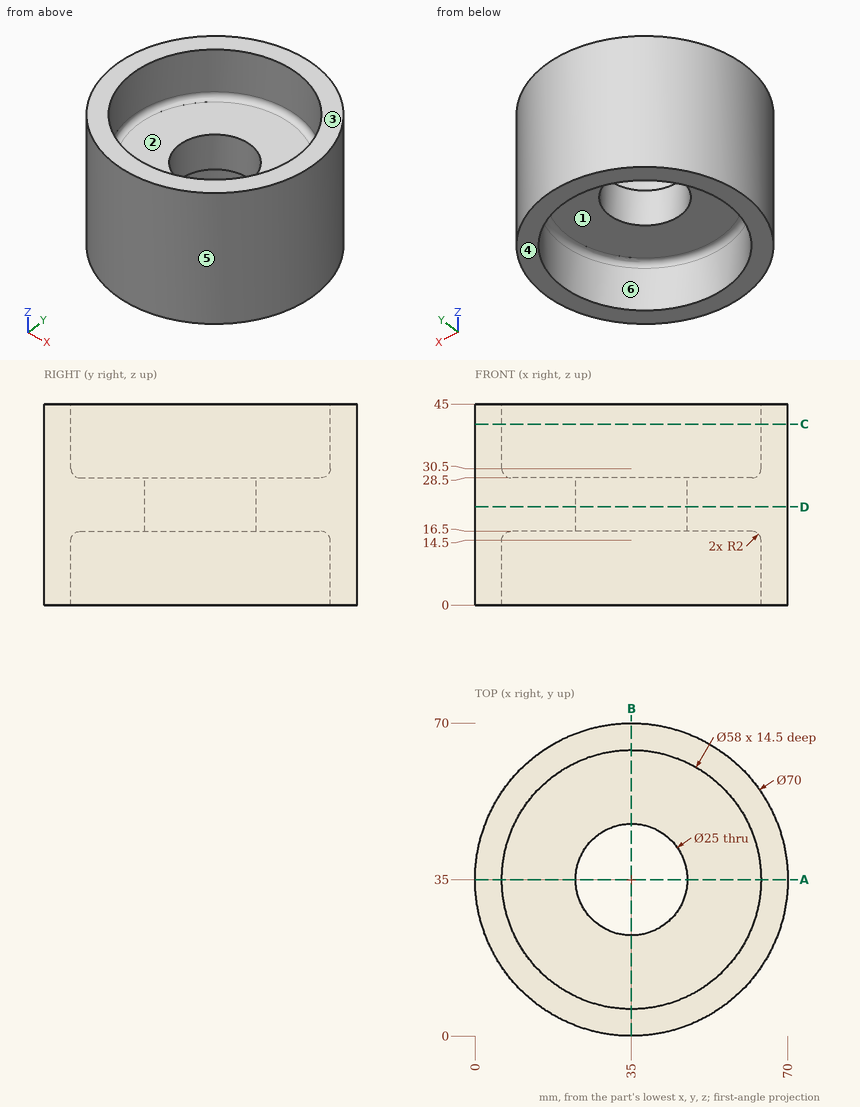
Could you check a few things on this drawing? It's one solid part, dimensions in mm from its lowest x, y, z. A direction names the side the tool comes from. Round coordinates to 2 decimals unless told otherwise and drop trailing zeros. Order: outer loops, then holes, each group sorted by start corner. A loop starts at its lowest first (then second) coordinate and runs counter-clockwise, first axis right, second up. Notation, with made-up numbers: M 82,46 L 115,46 A29 ccw 115,84 Z; hole C 59,-28.5 d6. An arc over 180 degrees is marked long. One line per question, with ' | ' between items. Start each with the question number.
(1) For P1, Ø10, axis at y = 19, z = 37, coming from the -X side; P2, Ø1, axis at x = 59.5, y = 31.5, coming from the -Z side; P3, Ø8, axis at y = 11, z = 8.5, coming from the +X side; P4, Ø3, axis at x = 46.5, y = 8.5, coming from the +Z side, each with a flat end and sliding along its axis, tell me the tip position at first contact or that it passes through.
(2) Suppose I cut it at D-D on z = 22. List the corners of the cut face in (x, y) for me, then the cut area to 3 significant figures.
(3) For the marked faces 1, 2 and 3, which set-ups out of +Z, -Z, +X, -X, +Y, -Y let a thin tool reach every point of the face, with its end or its side?
(4) Please list where these lines run through material, in increasing order: line 1 along Y through (x, z) = (35, 36); line 2 along X through (y, z) = (35, 19.5).
(5) Suppose I cut it at C-C on z = 40.5. List the corners of the cut face in (x, y) for me, then the cut area to 3 significant figures.
(6) Thinking about a two-plate mould opening in Y: for the marked faces 4, 5 and 6, which applies, +Y half, -Y half, draft (parallel to the pull), parting line (faces both ways), or undercut?
(7) Suppose I cut it at A-A on y = 35. List the corners of the cut face in (x, z) for me.
Geometry results:
1) P1: x = 1.77 | P2: z = 16.5 | P3: x = 63.72 | P4: z = 45
2) outline: C 35,35 d70; hole C 35,35 d25 | area: 3,360 mm²
3) face 1: -Z | face 2: +Z | face 3: +Z, +X, -X, +Y, -Y
4) line 1: 0 to 6, 64 to 70 | line 2: 0 to 22.5, 47.5 to 70
5) outline: C 35,35 d70; hole C 35,35 d58 | area: 1,210 mm²
6) face 4: draft | face 5: parting line | face 6: undercut
7) outline: M 0,0 L 6,0 L 6,14.5 A2 cw 8,16.5 L 22.5,16.5 L 22.5,28.5 L 8,28.5 A2 cw 6,30.5 L 6,45 L 0,45 Z; M 47.5,16.5 L 62,16.5 A2 cw 64,14.5 L 64,0 L 70,0 L 70,45 L 64,45 L 64,30.5 A2 cw 62,28.5 L 47.5,28.5 Z
